Work out the finished part from the listing and answer in its coordinate system (mm). Face numbers are marked on the shaded views. A direction names the side the tool comes from. Coordinates: 2 decimals unless noted, no trailing zeros. Loops run counter-clockwise (first coordinate to the right, second up) from the corner with the lowest first, then second, coordinate; pieces in that order, holes last. Notation, with made-up numbers: (44, 66.5) - (49, 66.5) arc R17 cw to (49, 87.5) - close; hole circle Ø3 at (64.5, 67.5). An arc over 180 degrees is marked (long way). Write each question's results on one line, items separated by ' | '. Start each with the question number.
Item 1: Section D-D, the plane x = 50 is taken. Write down the section's boundary in (y, z), plus the area to 3 significant figures.
Item 2: Section B-B, the plane y = 15 is taken. Write down the section's boundary in (x, z), plus the area to 3 significant figures.
Item 3: Section C-C, the plane z = 8.25 is taken. Write down the section's boundary in (x, y), plus the area to 3 significant figures.
Item 4: Each of these flat-tipped pins is pushed along its axis until it touches: pin 1 Ø5 at (x, z) = (41.5, 8) entering from -Y; pin 2 Ø6 at (x, y) = (73.5, 34.5) entering from +Z (3 decimals); pin 3 Ø1.5 at (x, z) = (46, 5.5) entering from -Y; pin 4 Ø3.5 at (x, z) = (89, 2) entering from +Y. Where does it stop, or does it pass through?
Item 5: Section A-A, the plane x = 73.5 is taken. Write down the section's boundary in (y, z), plus the area to 3 significant figures.
Item 6: Consider probe 1 along Z at (x, y) = (82, 6); probe 2 along Z at (x, y) = (51.5, 44); probe 3 along X at (y, z) = (49, 0.5). Determine where each line is inside the solid, lowest interval first. Write a range as [from, to].
Item 7: A tool of negligible diameter and unlimited length cuts with its end or side. For the marked faces 1 and 2, from which of +Z, -Z, +X, -X, +Y, -Y can it reach the whole face along a straight path? Write none if from no direction.
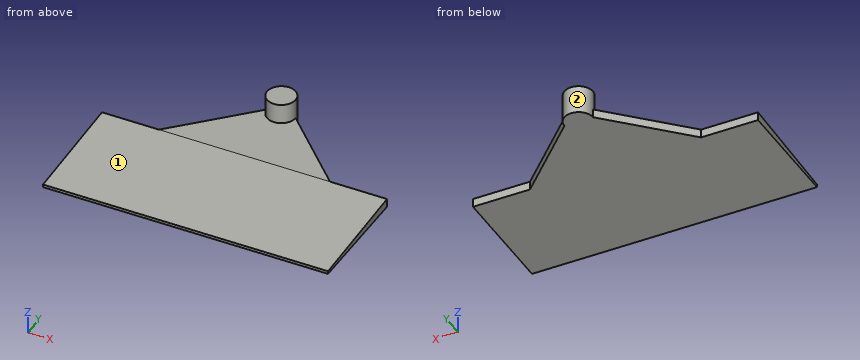
from build123d import *

# Parameters (mm, degrees)
F1_DEPTH = 100
F3_DEPTH = 3
F4_DEPTH = 10


with BuildPart() as f1:
    # F0 (on Right) → F1 (new body)
    with BuildSketch(Plane.YZ):
        Polygon((0, 1), (0, 0), (40, 0), (40, 3), align=None)
    extrude(amount=F1_DEPTH)

    # F2 (on face) → F3 (join)
    with BuildSketch(Plane(origin=(0, 0, 0), x_dir=(1, 0, 0), z_dir=(0, 0, -1))):
        with BuildLine():
            ThreePointArc((45, -65), (50, -60), (55, -65))
            Line((55, -65), (55, -40))
            Line((55, -40), (45, -40))
            Line((45, -40), (45, -65))
        make_face()
        Polygon((20, -40), (45, -65), (45, -40), align=None)
        Polygon((55, -40), (55, -65), (80, -40), align=None)
    extrude(amount=-F3_DEPTH)

    # F2 (on face) → F4 (join)
    with BuildSketch(Plane(origin=(0, 0, 0), x_dir=(1, 0, 0), z_dir=(0, 0, -1))):
        with BuildLine():
            Line((45, -65), (55, -65))
            ThreePointArc((55, -65), (50, -60), (45, -65))
        make_face()
        with BuildLine():
            ThreePointArc((45, -65), (50, -70), (55, -65))
            Line((55, -65), (45, -65))
        make_face()
    extrude(amount=-F4_DEPTH)


solid = f1.part
Answer key:
1) outline: (0, 0) - (70, 0) - (70, 10) - (60, 10) - (60, 3) - (40, 3) - (0, 1) - close | area: 240 mm^2
2) outline: (0, 0) - (100, 0) - (100, 1.75) - (0, 1.75) - close | area: 175 mm^2
3) outline: circle Ø10 at (50, 65) | area: 78.5 mm^2
4) pin 1: passes through | pin 2: stops at z = 2.875 | pin 3: stops at y = 61.2 | pin 4: stops at y = 40
5) outline: (0, 0) - (46.5, 0) - (46.5, 3) - (40, 3) - (0, 1) - close | area: 99.5 mm^2
6) probe 1: z = [0, 1.3] | probe 2: z = [0, 3] | probe 3: x = [29, 71]
7) face 1: +Z, +X, -X, -Y | face 2: +Z
